from build123d import *

# Parameters (mm, degrees)
SKETCH1_W            = 23.8
SKETCH1_H            = 3.2
BOSS_EXTRUDE1_DEPTH  = 15.8
SKETCH2_R            = 2.4
BOSS_EXTRUDE2_DEPTH  = 1.6
LPATTERN1_COUNT      = 2
LPATTERN1_PITCH      = 8
LPATTERN1_COUNT_DIR2 = 6
LPATTERN1_PITCH_DIR2 = 8
SHELL1_T             = -1.2
SKETCH3_R            = 3.25
SKETCH3_R_2          = 2.4
BOSS_EXTRUDE3_DEPTH  = 1.8
LPATTERN2_COUNT      = 2
LPATTERN2_PITCH      = 8


with BuildPart() as part:
    # Sketch1 → Boss-Extrude1 (new body)
    with BuildSketch(Plane.XY):
        with Locations((11.9, 1.6)):
            Rectangle(SKETCH1_W, SKETCH1_H)
    extrude(amount=-BOSS_EXTRUDE1_DEPTH)

    # Sketch2 → Boss-Extrude2 (add)
    with BuildSketch(Plane(origin=(0, 3.2, 0), x_dir=(1, 0, 0), z_dir=(0, 1, 0))):
        with Locations(Location((3.9, 3.9, 0), (0, 0, 270))):
            Circle(SKETCH2_R)
    boss_extrude2 = extrude(amount=BOSS_EXTRUDE2_DEPTH)

    # LPattern1: Boss-Extrude2 2 × 6, 6 skipped
    with Locations(*[(j * LPATTERN1_PITCH_DIR2, 0, -i * LPATTERN1_PITCH) for i in range(LPATTERN1_COUNT) for j in range(LPATTERN1_COUNT_DIR2) if (i, j) not in ((0, 0), (0, 3), (0, 4), (0, 5), (1, 3), (1, 4), (1, 5))]):
        add(boss_extrude2)

    # Shell1
    shell1_openings = [part.faces().sort_by_distance(p)[0] for p in [
        (11.9, 0, -7.9),
    ]]
    offset(amount=SHELL1_T, openings=shell1_openings, kind=Kind.INTERSECTION)

    # Sketch3 → Boss-Extrude3 (add)
    with BuildSketch(Plane.XZ.offset(-2)):
        with Locations(Location((7.9, -7.9, 0), (0, 0, 90))):
            Circle(SKETCH3_R)
        with Locations(Location((7.9, -7.9, 0), (0, 0, 270))):
            Circle(SKETCH3_R_2, mode=Mode.SUBTRACT)
    boss_extrude3 = extrude(amount=BOSS_EXTRUDE3_DEPTH)

    # LPattern2: Boss-Extrude3 ×2
    with Locations(*[(i * LPATTERN2_PITCH, 0, 0) for i in range(1, LPATTERN2_COUNT)]):
        add(boss_extrude3)


solid = part.part
Model file for the job. Use its own axes, mm. A direction names the side the tool comes from. Give positions to 0.01 mm unless a question says otherwise; leave off trailing zeros. Order: outer loops, then holes, each group sorted by start corner. A loop starts at its lowest first (then second) coordinate and runs counter-clockwise, first axis right, second up. Notation, with made-up numbers: (30.25, -4.5) - (37.25, -4.5) arc R6 cw to (37.25, 0.5) - close; hole circle Ø11 at (39, -35). An arc over 180 degrees is marked (long way). Write item = value, one per line. Start each with the question number.
1. Probe line 1 along Z through (x, y) = (12, 2.65); line 2 along X through (y, z) = (2.4, -11.9); line 3 along X through (y, z) = (3.25, -11.9). List the from-to ranges inside material, lowest first.
2. Which spindle directions (+Z, -Z, +X, -X, +Y, -Y) get a long thin tool onto all of the face, cutting with end or side? Do faces 1 (the cylindrical face through (14.28, 3.99, -12.21)), 2 (the flat face through (8, 2, -8)), 3 (the flat face through (12, 4.8, -4)). Say none if no direction does.
3. Two-plate mould, pull along X, no slides. Class faces 4 (the cylindrical face through (1.77, 3.99, -2.79)), 5 (the flat face through (4, 4.8, -4)), 6 (the cylindrical face through (1.557, 3.989, -12.42)): pulls with the +X half, pulls with the -X half, needs draft (parallel to the pull), parting line crosses it, or undercut.
4. Cut at C-C, the plane y = 4.35. List the corners of the cut face in (x, z), and give its area (3 significant figures).
5. Drop flat-ended pins along their axis: P1, Ø2, axis at x = 19.9, z = -11.9, coming from the -Y side; P2, Ø2.5, axis at x = 12, z = -12, coming from the -Y side; P3, Ø2.5, axis at x = 9, z = -8.5, coming from the -Y side. Give the stop position or say it passes through.
6. Cut at A-A, the plane y = 0.75. List the corners of the cut face in (x, z).
7. Cut at B-B, the plane x = 3.9. List the corners of the cut face in (y, z).
Taken from the geometry:
q1.line_1 = -15.8 to -13.1, -10.7 to -5.1, -2.7 to 0
q1.line_2 = 0 to 2.7, 5.1 to 10.7, 13.1 to 18.7, 21.1 to 23.8
q1.line_3 = 1.5 to 2.7, 5.1 to 6.3, 9.5 to 10.7, 13.1 to 14.3, 17.5 to 18.7, 21.1 to 22.3
q2.face_1 = +Y
q2.face_2 = -Y
q2.face_3 = +Z, -Z, +X, -X, +Y
q3.face_4 = undercut
q3.face_5 = needs draft
q3.face_6 = undercut
q4.outline = circle Ø4.8 at (3.9, -11.9); circle Ø4.8 at (3.9, -3.9); circle Ø4.8 at (11.9, -11.9); circle Ø4.8 at (11.9, -3.9); circle Ø4.8 at (19.9, -11.9); circle Ø4.8 at (19.9, -3.9)
q4.area = 109 mm²
q5.P1 = 3.6
q5.P2 = 2
q5.P3 = 0.2
q6.outline = (0, -15.8) - (23.8, -15.8) - (23.8, 0) - (0, 0) - close; circle Ø6.5 at (7.9, -7.9); circle Ø6.5 at (15.9, -7.9); hole (1.2, -14.6) - (22.6, -14.6) - (22.6, -1.2) - (1.2, -1.2) - close; hole circle Ø4.8 at (7.9, -7.9); hole circle Ø4.8 at (15.9, -7.9)
q7.outline = (0, -15.8) - (3.2, -15.8) - (3.2, -14.3) - (4.8, -14.3) - (4.8, -9.5) - (3.2, -9.5) - (3.2, -6.3) - (4.8, -6.3) - (4.8, -1.5) - (3.2, -1.5) - (3.2, 0) - (0, 0) - (0, -1.2) - (2, -1.2) - (2, -2.7) - (3.6, -2.7) - (3.6, -5.1) - (2, -5.1) - (2, -10.7) - (3.6, -10.7) - (3.6, -13.1) - (2, -13.1) - (2, -14.6) - (0, -14.6) - close
